Input: part model. Units: mm. Frame: model coordinates. Face numbers are marked on the shaded views. A direction names the side the tool comes from. Round coordinates to 2 decimals unless told otherwise and drop trailing zeros. Loops run counter-clockwise (first coordinate to the right, second up) from the corner with the lowest first, then second, coordinate; pieces in that order, holes last. Notation, with made-up numbers: (36, 35.25) -> (52, 35.25) arc R9 ccw to (52, 40.25) -> close; hole circle Ø9 at (33.5, 8). An arc over 180 degrees is marked (long way). Answer in a Markdown table with one row per item. Add a question column.
Q1. Section B-B, the plane x = -13.5. Output: boundary loops of the cut face in (y, z), and give its area (3 significant figures).
Q2. Section C-C, the plane y = 7.5. Output: boundary loops of the cut face in (x, z).
Q3. Reachability of the marked faces 4, 5 and 6 from +Z, -Z, +X, -X, +Y, -Y: full face, straight path, thin tool, end or side. Return the list, or none.
Q4. Section D-D, the plane y = -13. Output: boundary loops of the cut face in (x, z).
Q5. Section A-A, the plane z = 6.25. Output: boundary loops of the cut face in (x, y), and give its area (3 significant figures).
Q6. Ray query, L1, parallel to X at y = 11, z = 19; L2, parallel to Z at x = 17.5, y = -11; L3, parallel to X at y = 12, z = 3.25. Return the intervals inside material, ascending. Write a range as from..to.
Q7. Mould query, pull axis X, two halves, no side actions, for the marked faces 1, 2 and 3. Classes: pulls with the +X half, pulls with the -X half, needs draft (parallel to the pull), parting line crosses it, or undercut.
Q8. Pin query (flat end, axial travel): pin 1 (8 mm diameter, centred on x = -1, z = 15.5, fed in from -Y); pin 2 (4.5 mm diameter, centred on y = 6.5, z = 13, fed in from +X); pin 3 (2 mm diameter, centred on x = -7.5, y = -14.5, fed in from +Z). Return the tip coordinate at first contact, or that it passes through.
```python
from build123d import *

# Parameters (mm, degrees)
BOSS_EXTRUDE1_DEPTH = 5
BOSS_EXTRUDE2_DEPTH = 20
SKETCH6_R           = 1.8
CUT_EXTRUDE3_DEPTH  = 6


with BuildPart() as part:
    # Sketch1 → Boss-Extrude1 (new body)
    with BuildSketch(Plane.XY):
        Polygon((14.31372549, -4.264705882), (34.31372549, -4.264705882), (34.31372549, -19.264705882), (-20.68627451, -19.264705882), (-20.68627451, -4.264705882), (-0.68627451, -4.264705882), (-0.68627451, 15.735294118), (14.31372549, 15.735294118), align=None)
    extrude(amount=BOSS_EXTRUDE1_DEPTH)

    # Sketch2 → Boss-Extrude2 (add)
    with BuildSketch(Plane(origin=(0, 0, 0), x_dir=(-1, 0, 0), z_dir=(0, 0, -1))):
        Polygon((0.68627451, 15.735294118), (4.68627451, 15.735294118), (4.68627451, -0.264705882), (6.079970528, -0.264705882), (20.68627451, -0.264705882), (20.68627451, -4.264705882), (0.68627451, -4.264705882), align=None)
    boss_extrude2 = extrude(amount=-BOSS_EXTRUDE2_DEPTH)

    # Mirror1: Boss-Extrude2 across plane
    add(boss_extrude2.mirror(Plane.ZY.offset(-6.81372549)))

    # Sketch6 → Cut-Extrude3 (cut, through all)
    with BuildSketch(Plane.XY.offset(5)):
        with Locations((6.81372549, 8.235294118)):
            Circle(SKETCH6_R)
        with Locations((-13.18627451, -11.764705882)):
            Circle(SKETCH6_R)
        with Locations((26.81372549, -11.764705882)):
            Circle(SKETCH6_R)
    extrude(amount=-CUT_EXTRUDE3_DEPTH, mode=Mode.SUBTRACT)


solid = part.part
```
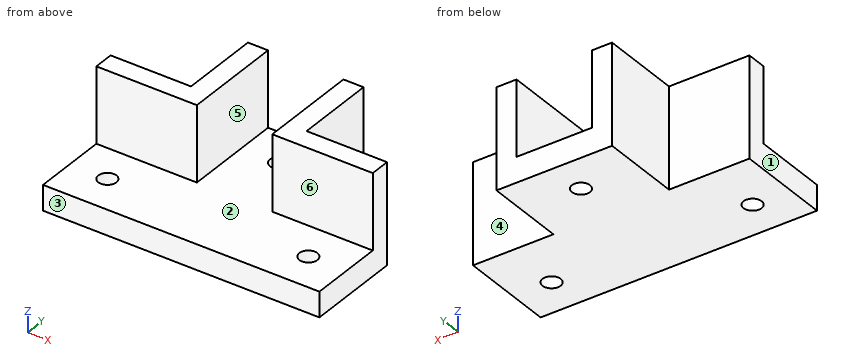
Answer block:
| question | item | result |
|---|---|---|
| 1 | outline | (-19.26, 0) -> (-13.54, 0) -> (-13.54, 5) -> (-19.26, 5) -> close; (-9.99, 0) -> (-0.26, 0) -> (-0.26, 20) -> (-4.26, 20) -> (-4.26, 5) -> (-9.99, 5) -> close |
| 1 | area | 137 mm^2 |
| 2 | outline | (-4.69, 0) -> (5.17, 0) -> (5.17, 5) -> (-0.69, 5) -> (-0.69, 20) -> (-4.69, 20) -> close; (8.46, 0) -> (18.31, 0) -> (18.31, 20) -> (14.31, 20) -> (14.31, 5) -> (8.46, 5) -> close |
| 3 | face 4 | +Z, -Z, +X, +Y |
| 3 | face 5 | +Z, +Y, -Y |
| 3 | face 6 | +Z, +X, -X, -Y |
| 4 | outline | (-20.69, 0) -> (-14.5, 0) -> (-14.5, 5) -> (-20.69, 5) -> close; (-11.88, 0) -> (25.5, 0) -> (25.5, 5) -> (-11.88, 5) -> close; (28.12, 0) -> (34.31, 0) -> (34.31, 5) -> (28.12, 5) -> close |
| 5 | outline | (-20.69, -4.26) -> (-0.69, -4.26) -> (-0.69, 15.74) -> (-4.69, 15.74) -> (-4.69, -0.26) -> (-20.69, -0.26) -> close; (14.31, -4.26) -> (34.31, -4.26) -> (34.31, -0.26) -> (18.31, -0.26) -> (18.31, 15.74) -> (14.31, 15.74) -> close |
| 5 | area | 288 mm^2 |
| 6 | L1 | -4.69..-0.69, 14.31..18.31 |
| 6 | L2 | 0..5 |
| 6 | L3 | -4.69..18.31 |
| 7 | face 1 | pulls with the -X half |
| 7 | face 2 | undercut |
| 7 | face 3 | needs draft |
| 8 | pin 1 | y = -4.26 |
| 8 | pin 2 | x = 18.31 |
| 8 | pin 3 | z = 5 |
